```python
from build123d import *

# Parameters (mm, degrees)
BOSS_EXTRUDE1_DEPTH = 3
SKETCH3_W           = 166.2
SKETCH3_H           = 58
BOSS_EXTRUDE2_DEPTH = 20
SKETCH4_R           = 1.75
CUT_EXTRUDE1_DEPTH  = 205.768161588
FILLET1_R           = 4
FILLET2_R           = 3
CUT_EXTRUDE2_REACH  = 207.441
SKETCH5_R           = 2
SKETCH6_R           = 1.75
CUT_EXTRUDE3_DEPTH  = 205.768161588
SKETCH8_R           = 1.75
CUT_EXTRUDE5_DEPTH  = 205.768161588


with BuildPart() as part:
    # Sketch2 → Boss-Extrude1 (new, symmetric)
    with BuildSketch(Plane.XY):
        Polygon((-187, 22.75), (-187, -22.75), (-107, -22.75), (-107, -81), (113, -81), (113, -22.75), (187, -22.75), (187, 22.75), (113, 22.75), (113, 81), (-107, 81), (-107, 22.75), align=None)
    extrude(amount=BOSS_EXTRUDE1_DEPTH, both=True)

    # Sketch3 → Boss-Extrude2 (add)
    with BuildSketch(Plane.XY.offset(3)):
        Polygon((-187, -1.5), (-90, -1.5), (-90, -32), (82.2, -32), (82.2, -1.5), (187, -1.5), (187, 1.5), (82.2, 1.5), (82.2, 32), (-90, 32), (-90, 1.5), (-187, 1.5), align=None)
        with Locations((-3.9, 0)):
            Rectangle(SKETCH3_W, SKETCH3_H, mode=Mode.SUBTRACT)
    extrude(amount=BOSS_EXTRUDE2_DEPTH)

    # Sketch4 → Cut-Extrude1 (cut, through all)
    with BuildSketch(Plane.XY.offset(3)):
        with Locations((-36.6, -67)):
            Circle(SKETCH4_R)
        with Locations((-67, -51)):
            Circle(SKETCH4_R)
        with Locations((13.4, -67)):
            Circle(SKETCH4_R)
        with Locations((-17, -51)):
            Circle(SKETCH4_R)
        with Locations((63.4, -67)):
            Circle(SKETCH4_R)
        with Locations((33, -51)):
            Circle(SKETCH4_R)
        with Locations(Location((33, 51, 0), (0, 0, 180))):
            Circle(SKETCH4_R)
        with Locations(Location((63.4, 67, 0), (0, 0, 180))):
            Circle(SKETCH4_R)
        with Locations(Location((-17, 51, 0), (0, 0, 180))):
            Circle(SKETCH4_R)
        with Locations(Location((13.4, 67, 0), (0, 0, 180))):
            Circle(SKETCH4_R)
        with Locations(Location((-67, 51, 0), (0, 0, 180))):
            Circle(SKETCH4_R)
        with Locations(Location((-36.6, 67, 0), (0, 0, 180))):
            Circle(SKETCH4_R)
    extrude(amount=-CUT_EXTRUDE1_DEPTH, mode=Mode.SUBTRACT)

    # Fillet1
    fillet1_edges = [part.edges().sort_by_distance(p)[0] for p in [
        (-107, -22.75, 0),
        (-107, 22.75, 0),
        (113, 22.75, 0),
        (113, -22.75, 0),
    ]]
    fillet(fillet1_edges, radius=FILLET1_R)

    # Fillet2
    fillet2_edges = [part.edges().sort_by_distance(p)[0] for p in [
        (-87, 0, 3),
        (-3.9, -29, 3),
        (79.2, 0, 3),
        (-3.9, 29, 3),
        (-138.5, -1.5, 3),
        (-90, -16.75, 3),
        (-3.9, -32, 3),
        (82.2, -16.75, 3),
        (134.6, -1.5, 3),
        (134.6, 1.5, 3),
        (82.2, 16.75, 3),
        (-3.9, 32, 3),
        (-90, 16.75, 3),
        (-138.5, 1.5, 3),
    ]]
    fillet(fillet2_edges, radius=FILLET2_R)

    # Sketch5 → Cut-Extrude2 (cut, up to next)
    with BuildSketch(Plane(origin=(0, 0, -3), x_dir=(-1, 0, 0), z_dir=(0, 0, -1)), mode=Mode.PRIVATE) as cut_extrude2_sk1:
        with Locations((-103, -12.75)):
            Circle(SKETCH5_R)
    cut_extrude2_tool1 = extrude(cut_extrude2_sk1.sketch, amount=-CUT_EXTRUDE2_REACH, mode=Mode.PRIVATE) & part.part
    # Sketch5 → Cut-Extrude2 (cut, up to next)
    with BuildSketch(Plane(origin=(0, 0, -3), x_dir=(-1, 0, 0), z_dir=(0, 0, -1)), mode=Mode.PRIVATE) as cut_extrude2_sk2:
        with Locations((-103, 12.75)):
            Circle(SKETCH5_R)
    cut_extrude2_tool2 = extrude(cut_extrude2_sk2.sketch, amount=-CUT_EXTRUDE2_REACH, mode=Mode.PRIVATE) & part.part
    # Sketch5 → Cut-Extrude2 (cut, up to next)
    with BuildSketch(Plane(origin=(0, 0, -3), x_dir=(-1, 0, 0), z_dir=(0, 0, -1)), mode=Mode.PRIVATE) as cut_extrude2_sk3:
        with Locations((-179, 12.75)):
            Circle(SKETCH5_R)
    cut_extrude2_tool3 = extrude(cut_extrude2_sk3.sketch, amount=-CUT_EXTRUDE2_REACH, mode=Mode.PRIVATE) & part.part
    # Sketch5 → Cut-Extrude2 (cut, up to next)
    with BuildSketch(Plane(origin=(0, 0, -3), x_dir=(-1, 0, 0), z_dir=(0, 0, -1)), mode=Mode.PRIVATE) as cut_extrude2_sk4:
        with Locations((-179, -12.75)):
            Circle(SKETCH5_R)
    cut_extrude2_tool4 = extrude(cut_extrude2_sk4.sketch, amount=-CUT_EXTRUDE2_REACH, mode=Mode.PRIVATE) & part.part
    # Sketch5 → Cut-Extrude2 (cut, up to next)
    with BuildSketch(Plane(origin=(0, 0, -3), x_dir=(-1, 0, 0), z_dir=(0, 0, -1)), mode=Mode.PRIVATE) as cut_extrude2_sk5:
        with Locations((177, 12.75)):
            Circle(SKETCH5_R)
    cut_extrude2_tool5 = extrude(cut_extrude2_sk5.sketch, amount=-CUT_EXTRUDE2_REACH, mode=Mode.PRIVATE) & part.part
    # Sketch5 → Cut-Extrude2 (cut, up to next)
    with BuildSketch(Plane(origin=(0, 0, -3), x_dir=(-1, 0, 0), z_dir=(0, 0, -1)), mode=Mode.PRIVATE) as cut_extrude2_sk6:
        with Locations((177, -12.75)):
            Circle(SKETCH5_R)
    cut_extrude2_tool6 = extrude(cut_extrude2_sk6.sketch, amount=-CUT_EXTRUDE2_REACH, mode=Mode.PRIVATE) & part.part
    # Sketch5 → Cut-Extrude2 (cut, up to next)
    with BuildSketch(Plane(origin=(0, 0, -3), x_dir=(-1, 0, 0), z_dir=(0, 0, -1)), mode=Mode.PRIVATE) as cut_extrude2_sk7:
        with Locations((101, -12.75)):
            Circle(SKETCH5_R)
    cut_extrude2_tool7 = extrude(cut_extrude2_sk7.sketch, amount=-CUT_EXTRUDE2_REACH, mode=Mode.PRIVATE) & part.part
    # Sketch5 → Cut-Extrude2 (cut, up to next)
    with BuildSketch(Plane(origin=(0, 0, -3), x_dir=(-1, 0, 0), z_dir=(0, 0, -1)), mode=Mode.PRIVATE) as cut_extrude2_sk8:
        with Locations((101, 12.75)):
            Circle(SKETCH5_R)
    cut_extrude2_tool8 = extrude(cut_extrude2_sk8.sketch, amount=-CUT_EXTRUDE2_REACH, mode=Mode.PRIVATE) & part.part
    add(cut_extrude2_tool1.solids().sort_by_distance((103, -12.75, -3))[0], mode=Mode.SUBTRACT)
    add(cut_extrude2_tool2.solids().sort_by_distance((103, 12.75, -3))[0], mode=Mode.SUBTRACT)
    add(cut_extrude2_tool3.solids().sort_by_distance((179, 12.75, -3))[0], mode=Mode.SUBTRACT)
    add(cut_extrude2_tool4.solids().sort_by_distance((179, -12.75, -3))[0], mode=Mode.SUBTRACT)
    add(cut_extrude2_tool5.solids().sort_by_distance((-177, 12.75, -3))[0], mode=Mode.SUBTRACT)
    add(cut_extrude2_tool6.solids().sort_by_distance((-177, -12.75, -3))[0], mode=Mode.SUBTRACT)
    add(cut_extrude2_tool7.solids().sort_by_distance((-101, -12.75, -3))[0], mode=Mode.SUBTRACT)
    add(cut_extrude2_tool8.solids().sort_by_distance((-101, 12.75, -3))[0], mode=Mode.SUBTRACT)

    # Sketch6 → Cut-Extrude3 (cut, through all)
    with BuildSketch(Plane.XY.offset(3)):
        with Locations((-51.8, -76)):
            Circle(SKETCH6_R)
        with Locations(Location((-51.8, -42, 0), (0, 0, 180))):
            Circle(SKETCH6_R)
        with Locations((-1.8, -76)):
            Circle(SKETCH6_R)
        with Locations(Location((-1.8, -42, 0), (0, 0, 180))):
            Circle(SKETCH6_R)
        with Locations((48.2, -76)):
            Circle(SKETCH6_R)
        with Locations(Location((48.2, -42, 0), (0, 0, 180))):
            Circle(SKETCH6_R)
        with Locations((48.2, 42)):
            Circle(SKETCH6_R)
        with Locations(Location((48.2, 76, 0), (0, 0, 180))):
            Circle(SKETCH6_R)
        with Locations((-1.8, 42)):
            Circle(SKETCH6_R)
        with Locations(Location((-1.8, 76, 0), (0, 0, 180))):
            Circle(SKETCH6_R)
        with Locations((-51.8, 42)):
            Circle(SKETCH6_R)
        with Locations(Location((-51.8, 76, 0), (0, 0, 180))):
            Circle(SKETCH6_R)
    extrude(amount=-CUT_EXTRUDE3_DEPTH, mode=Mode.SUBTRACT)

    # Sketch8 → Cut-Extrude5 (cut, through all)
    with BuildSketch(Plane.XY.offset(3)):
        with Locations((-80.9, -16)):
            Circle(SKETCH8_R)
        with Locations(Location((-80.9, 16, 0), (0, 0, 180))):
            Circle(SKETCH8_R)
        with Locations((73.1, 16)):
            Circle(SKETCH8_R)
        with Locations(Location((73.1, -16, 0), (0, 0, 180))):
            Circle(SKETCH8_R)
    extrude(amount=-CUT_EXTRUDE5_DEPTH, mode=Mode.SUBTRACT)


solid = part.part
```
The model under review builds one solid part; all positions refer to its coordinate system, in mm. A direction names the side the tool comes from. Coordinates: 2 decimals unless noted, no trailing zeros. Write each loop counter-clockwise with the first axis right and the second up, starting at its lowest first coordinate (ties: lowest second). Pieces come first, ordered by that corner, then holes. Notation, with made-up numbers: (-24, -39) - (22, -39) arc R16 ccw to (22, -19) - close; hole circle Ø9 at (-15, 74). An arc over 180 degrees is marked (long way). Answer in a Markdown table with one row per item. Add a question column.
Q1. Consider section A-A on z = 14.75. Give the boundary of the cut face in (x, y), then the cut area to 3 significant figures.
Q2. Draft analysis for pull direction Y (two halves, no side actions). For faces 4 (the face through (-90, -17, 14)), 5 (the face through (-87, 0, 14)), 6 (the face through (-3, 32, 14)), state which applies: +Y half, -Y half, draft (parallel to the pull), parting line (faces both ways), or undercut.
Q3. Clearance check with flat-ended pins moving along their axes: pin 1 (8.5 mm diameter, centred on y = 17.5, z = 18.5, fed in from -X); pin 2 (6.5 mm diameter, centred on x = 155.5, z = -1.5, fed in from -Y); pin 3 (2 mm diameter, centred on x = -3, z = 12.5, fed in from -Y); pin 4 (2.5 mm diameter, centred on x = -177, y = -12.75, fed in from -Z). State where each tip first meets the part, or that it passes through.
Q4. To check wall thickness, follow line 1 along X through (y, z) = (-67, 1.45); line 2 along Y through (x, z) = (-51.8, 0.3); line 3 along Y through (x, z) = (-67, 0.9). State the ranges of each line that lie inside material, in increasing order. Write a range as from..to.
Q5. For faces 1 (the face through (-3, 52, 3)), 2 (the face through (-5, 0, 3)), 3 (the face through (-5, -32, 14)), list the 3-axis set-ups (+Z, -Z, +X, -X, +Y, -Y) from which the entire face can be reached by the end or side of a thin tool; tool diameter is ignored.
Q6. Consider section B-B on y = -60.5. Give the boundary of the cut face in (x, z), then the cut area to 3 significant figures.
Answers below:
| question | item | result |
|---|---|---|
| 1 | outline | (-187, -1.5) - (-90, -1.5) - (-90, -32) - (82.2, -32) - (82.2, -1.5) - (187, -1.5) - (187, 1.5) - (82.2, 1.5) - (82.2, 32) - (-90, 32) - (-90, 1.5) - (-187, 1.5) - close; hole (-87, -29) - (79.2, -29) - (79.2, 29) - (-87, 29) - close |
| 1 | area | 1,990 mm² |
| 2 | face 4 | draft |
| 2 | face 5 | undercut |
| 2 | face 6 | +Y half |
| 3 | pin 1 | x = -90 |
| 3 | pin 2 | y = -22.75 |
| 3 | pin 3 | y = -32 |
| 3 | pin 4 | through |
| 4 | line 1 | -107..-38.35, -34.85..11.65, 15.15..61.65, 65.15..113 |
| 4 | line 2 | -81..-77.75, -74.25..-43.75, -40.25..40.25, 43.75..74.25, 77.75..81 |
| 4 | line 3 | -81..-52.75, -49.25..49.25, 52.75..81 |
| 5 | face 1 | +Z, +Y |
| 5 | face 2 | +Z |
| 5 | face 3 | +Z, +X, -X, -Y |
| 6 | outline | (-107, -3) - (113, -3) - (113, 3) - (-107, 3) - close |
| 6 | area | 1,320 mm² |
